Verification items for the finished model (mm, model axes). A direction names the side the tool comes from. Round coordinates to 2 decimals unless told otherwise and drop trailing zeros. Order: outer loops, then holes, each group sorted by start corner. A loop starts at its lowest first (then second) coordinate and runs counter-clockwise, first axis right, second up. Notation, with made-up numbers: M 5,-33 L 54,-33 A15 ccw 54,-17 Z; hole C 76,86.5 d9. An arc over 180 degrees is marked long. Use CSV: the item, a comma, the result in double quotes. Start each with the question number.
Q1. Sectioned sample at B-B (y = 82.5). Enter the section's corners in (x, z).
Q2. Scan lines: line 1 (X direction, y = 74.6, z = 0); line 2 (Z direction, x = 5, y = 75); line 3 (Y direction, x = -15, z = 11.5). Record each from-to range of solid material in increasing order.
Q3. Gauge pin test, flat ends, axial feed: pin 1 Ø5 at (x, z) = (-13, -11) entering from +Y; pin 2 Ø0.8 at (x, z) = (11, 0) entering from -Y; pin 3 Ø3 at (x, z) = (6, -9) entering from -Y. Record the tip position at first contact, or that the pin passes through.
Q4. Set-up check for faces 1 (the face through (6, 73.5, -10)), 2 (the face through (0, 0, 0)), 3 (the face through (-4.5, 13.5, 4.5)): record each of +Z, -Z, +X, -X, +Y, -Y from which the full face is reachable in a straight line by a thin tool's end or side.
Q5. Mould release check, pull along Z, two halves, no side actions. Record for faces 4 (the face through (-1.802, 12.74, -5.723)), 5 (the face through (-6.26, 14.98, 10.52)), 6 (the face through (0, 94, 0)): +Z half, -Z half, draft (parallel to the pull), parting line (faces both ways), or undercut.
Q6. Sectioned sample at C-C (y = 40.5). Enter the section's corners in (x, z).
Q7. Sectioned sample at A-A (x = -11). Enter the section's corners in (y, z).
Q8. Sectioned sample at D-D (x = 8). Enter the section's corners in (y, z), and give its area (3 significant figures).
```python
from build123d import *

# Parameters (mm, degrees)
ESQUISSE2_R             = 1.25
ENL_V_MAT_EXTRU_1_DEPTH = 3
ENL_V_START             = -60
ESQUISSE2_2_R           = 1.25
ENL_V_MAT_EXTRU_2_DEPTH = 3
CHANFREIN1_SIZE         = 0.5


with BuildPart() as part:
    # Esquisse1 → Révolution1 (revolve)
    with BuildSketch(Plane.XY, mode=Mode.PRIVATE) as r_volution1_sk:
        Polygon((0, 0), (0, 94), (3, 94), (3, 78), (6, 78), (6, 76.5), (19, 76.5), (19, 13.5), (6, 13.5), (6, 12), (3, 12), (3, 0), align=None)
    revolve(r_volution1_sk.sketch.rotate(Axis((0, 0, 0), (0, 1, 0)), 90), axis=Axis((0, 0, 0), (0, 1, 0)))

    # Esquisse2 → Enlèv. mat.-Extru.1 (cut)
    with BuildSketch(Plane.XZ.offset(-13.5)):
        with Locations(Location((11, 0, 0), (0, 0, 270))):
            Circle(ESQUISSE2_R)
        with Locations(Location((5.5, -9.526279442, 0), (0, 0, 270))):
            Circle(ESQUISSE2_R)
        with Locations(Location((-5.5, -9.526279442, 0), (0, 0, 270))):
            Circle(ESQUISSE2_R)
        with Locations(Location((-11, 0, 0), (0, 0, 270))):
            Circle(ESQUISSE2_R)
        with Locations(Location((-5.5, 9.526279442, 0), (0, 0, 270))):
            Circle(ESQUISSE2_R)
        with Locations(Location((5.5, 9.526279442, 0), (0, 0, 270))):
            Circle(ESQUISSE2_R)
    extrude(amount=-ENL_V_MAT_EXTRU_1_DEPTH, mode=Mode.SUBTRACT)

    # Esquisse2<2> → Enlèv. mat.-Extru.2 (cut)
    with BuildSketch(Plane.XZ.offset(-13.5).offset(ENL_V_START)):
        with Locations(Location((11, 0, 0), (0, 0, 270))):
            Circle(ESQUISSE2_2_R)
        with Locations(Location((5.5, -9.526279442, 0), (0, 0, 270))):
            Circle(ESQUISSE2_2_R)
        with Locations(Location((-5.5, -9.526279442, 0), (0, 0, 270))):
            Circle(ESQUISSE2_2_R)
        with Locations(Location((-11, 0, 0), (0, 0, 270))):
            Circle(ESQUISSE2_2_R)
        with Locations(Location((-5.5, 9.526279442, 0), (0, 0, 270))):
            Circle(ESQUISSE2_2_R)
        with Locations(Location((5.5, 9.526279442, 0), (0, 0, 270))):
            Circle(ESQUISSE2_2_R)
    extrude(amount=-ENL_V_MAT_EXTRU_2_DEPTH, mode=Mode.SUBTRACT)

    # Chanfrein1
    chanfrein1_edges = [part.edges().sort_by_distance(p)[0] for p in [
        (0, 94, 3),
        (0, 0, 3),
    ]]
    chamfer(chanfrein1_edges, length=CHANFREIN1_SIZE)


solid = part.part
```
Verdict:
1,outline,"C 0,0 d6"
2,line 1,"x = -19 to -12.25, -9.75 to 9.75, 12.25 to 19"
2,line 2,"z = -18.33 to -10.67, -8.38 to 8.38, 10.67 to 18.33"
2,line 3,"y = 13.5 to 76.5"
3,pin 1,"stops at y = 76.5"
3,pin 2,"stops at y = 16.5"
3,pin 3,"stops at y = 13.5"
4,face 1,"+Y"
4,face 2,"+Z, -Z, +X, -X, -Y"
4,face 3,"-Y"
5,face 4,"parting line"
5,face 5,"undercut"
5,face 6,"draft"
6,outline,"C 0,0 d38"
7,outline,"M 13.5,-15.49 L 76.5,-15.49 L 76.5,-1.25 L 73.5,-1.25 L 73.5,1.25 L 76.5,1.25 L 76.5,15.49 L 13.5,15.49 L 13.5,1.25 L 16.5,1.25 L 16.5,-1.25 L 13.5,-1.25 Z"
8,outline,"M 13.5,-17.23 L 76.5,-17.23 L 76.5,17.23 L 13.5,17.23 Z"
8,area,"2,170 mm²"
